Could you check a few things on this drawing? It's one solid part, dimensions in mm from its lowest x, y, z. A direction names the side the tool comes from. Give positions to 0.01 mm unless a question says otherwise; leave off trailing zeros. Loops run counter-clockwise (first coordinate to the right, second up) from the corner with the lowest first, then second, coordinate; pieces in that order, holes last. Notation, with made-up numbers: (9.5, 14.5) - (22.5, 14.5) arc R22 ccw to (22.5, 32.5) - close; hole circle Ø4 at (70.5, 47.25). An arc over 180 degrees is marked (long way). Use CSV: the item, a comma, the result in double quotes.
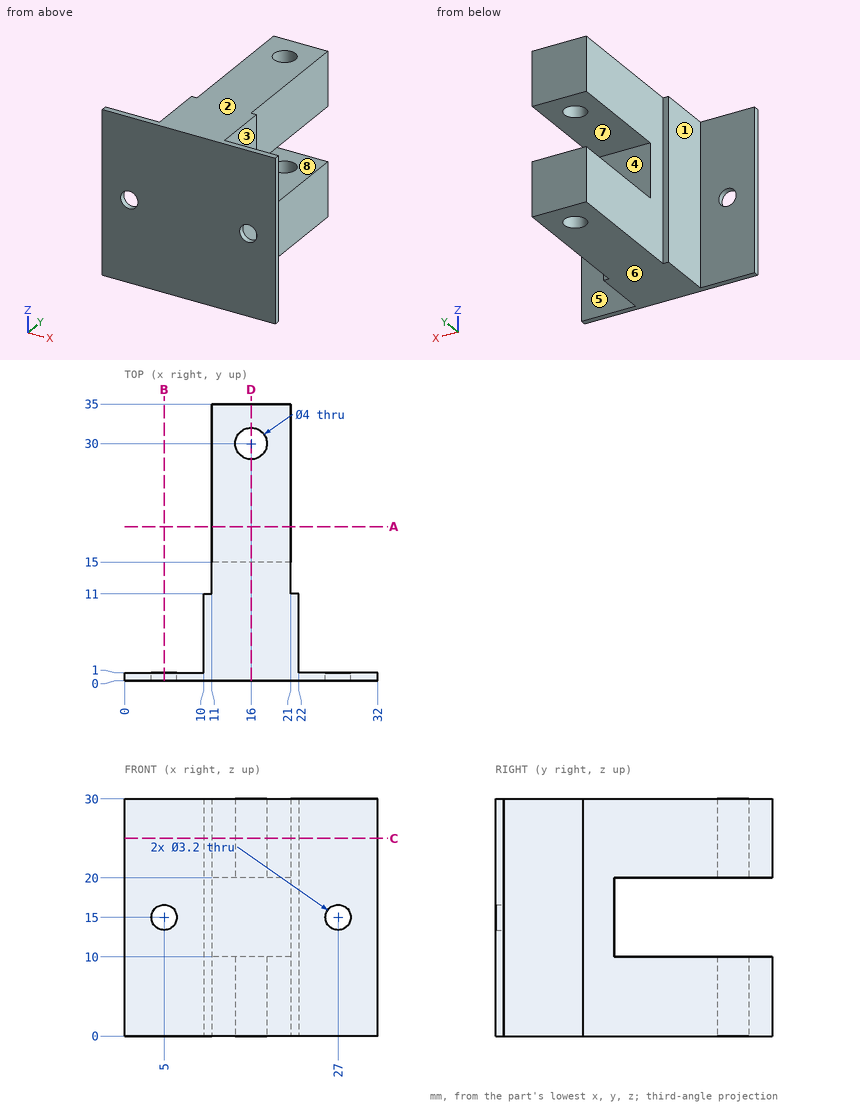
1) I'm going to push flat-ended pins straight in: P1, Ø8, axis at y = 26, z = 21, coming from the -X side; P2, Ø5, axis at x = 24.5, y = 23.5, coming from the +Z side; P3, Ø5, axis at x = 27, z = 7, coming from the +Y side; P4, Ø0.5, axis at x = 21.5, z = 15.5, coming from the +Y side. Where does each tip first touch, or does it pass through?
Answer below:
P1,"stops at x = 11"
P2,"passes through"
P3,"stops at y = 1"
P4,"stops at y = 11"
2) Which directions (+Z, -Z, +X, -X, +Y, -Y) give clear straight access to the entire face, cutting with the end or side of a thin tool? Please do the marked faces 1, 2, 3 and 4.
Answer below:
face 1,"+Z, -Z, -X, +Y"
face 2,"+Z, +X, -X, +Y, -Y"
face 3,"+Z, -Z, +X, +Y"
face 4,"+X, -X, +Y"
3) Suppose I cut it at A-A (y = 19.5). Please give me the cut outline in (x, z).
Answer below:
outline,"(11, 0) - (21, 0) - (21, 10) - (11, 10) - close; (11, 20) - (21, 20) - (21, 30) - (11, 30) - close"
4) Suppose I cut it at B-B (x = 5). Please give me the cut outline in (y, z).
Answer below:
outline,"(0, 0) - (1, 0) - (1, 13.4) - (0, 13.4) - close; (0, 16.6) - (1, 16.6) - (1, 30) - (0, 30) - close"
5) I need wall thicknesses on line 1 along X through (y, z) = (0.25, 15); line 2 along Y through (x, z) = (16, 23.25); line 3 along Z through (x, y) = (27, 0.35). Which ranges of each line are inside material? Lowest first, please.
Answer below:
line 1,"x = 0 to 3.4, 6.6 to 25.4, 28.6 to 32"
line 2,"y = 0 to 28, 32 to 35"
line 3,"z = 0 to 13.4, 16.6 to 30"
6) Suppose I cut it at C-C (z = 25). Please give me the cut outline in (x, y), plus the area to 3 significant figures.
Answer below:
outline,"(0, 0) - (32, 0) - (32, 1) - (22, 1) - (22, 11) - (21, 11) - (21, 35) - (11, 35) - (11, 11) - (10, 11) - (10, 1) - (0, 1) - close; hole circle Ø4 at (16, 30)"
area,"379 mm2"
7) We'd pull the mould along Z, two halves only. Please class the marked faces 5, 6, 7 and 8: +Z half, -Z half, draft (parallel to the pull), parting line (faces both ways), or undercut.
Answer below:
face 5,"draft"
face 6,"-Z half"
face 7,"undercut"
face 8,"undercut"
8) Suppose I cut it at D-D (x = 16). Please give me the cut outline in (y, z).
Answer below:
outline,"(0, 0) - (28, 0) - (28, 10) - (15, 10) - (15, 20) - (28, 20) - (28, 30) - (0, 30) - close; (32, 0) - (35, 0) - (35, 10) - (32, 10) - close; (32, 20) - (35, 20) - (35, 30) - (32, 30) - close"
